Autodesk Fusion 360 part; units mm, degrees
sketch "Sketch2" plane through (0, 0, 0) normal (0, 0, 1) x (1, 0, 0)
  line L0 (-21.3111, -3.5) -> (-24.01, -3.5)
  line L1 (-27.5, -0.01) -> (-27.5, 0.01)
  line L2 (-24.01, 3.5) -> (-21.3111, 3.5)
  line L3 (27.5, 0.01) -> (27.5, -0.01)
  arc A0 (-27.5, -0.01) -> (-24.01, -3.5) centre (-24.01, -0.01) ccw
  arc A1 (-24.01, 3.5) -> (-27.5, 0.01) centre (-24.01, 0.01) ccw
  arc A2 (27.5, 0.01) -> (24.01, 3.5) centre (24.01, 0.01) ccw
  arc A3 (24.01, -3.5) -> (27.5, -0.01) centre (24.01, -0.01) ccw
  circle A4 centre (24, 0) radius 2.5
  circle A5 centre (-24, 0) radius 2.5
  circle A6 centre (6.7175, 6.7175) radius 1.65
  circle A7 centre (-5.6569, 5.6569) radius 1.65
  circle A8 centre (-6.7175, -6.7175) radius 1.65
  circle A9 centre (5.6569, -5.6569) radius 1.65
  circle A10 centre (0, 0) radius 12.5
  line L4 (-17.9244, 4.3738) -> (-6.0478, 10.9396)
  line L5 (-17.9244, -4.3738) -> (-6.0478, -10.9396)
  line L6 (17.9244, 4.3738) -> (6.0478, 10.9396)
  line L7 (17.9244, -4.3738) -> (6.0478, -10.9396)
  arc A11 (-21.3111, 3.5) -> (-17.9244, 4.3738) centre (-21.3111, 10.5) ccw
  arc A12 (-17.9244, -4.3738) -> (-21.3111, -3.5) centre (-21.3111, -10.5) ccw
  line L8 (24.01, 3.5) -> (21.3111, 3.5)
  line L9 (24.01, -3.5) -> (21.3111, -3.5)
  arc A13 (21.3111, -3.5) -> (17.9244, -4.3738) centre (21.3111, -10.5) ccw
  arc A14 (17.9244, 4.3738) -> (21.3111, 3.5) centre (21.3111, 10.5) ccw
  line L10 (21.3111, -3.5) -> (12, -3.5)
  line L11 (-12, -3.5) -> (-21.3111, -3.5)
  line L12 (-21.3111, 3.5) -> (-12, 3.5)
  line L13 (12, 3.5) -> (21.3111, 3.5)
  line L14 (-16.3799, 2.0847) -> (-27.5, 3.5) construction
  line L15 (-27.5, -3.5) -> (-16.3799, -2.0847) construction
  line L16 (-12.4, -1.5782) -> (12.4, 1.5782) construction
  line L17 (25.3613, 3.2278) -> (27.5, 3.5) construction
  line L18 (27.5, -3.5) -> (25.3613, -3.2278) construction
  line L19 (12.4, -1.5782) -> (-12.4, 1.5782) construction
  circle A15 centre (-16.01, 0.01) radius 2.5
  circle A16 centre (16, 0) radius 2.5
  dimension "d42" = 9.5
  dimension "d44" = 8
  dimension "d45" = 8
  dimension "d46" = 9.5
  dimension "d47" = 55
  dimension "d48" = 7
  dimension "d49" = 3.49
  dimension "d50" = 3.49
  dimension "d51" = 3.49
  dimension "d52" = 3.49
  dimension "d53" = 24
  dimension "d54" = 5
  dimension "d55" = 24
  dimension "d56" = 5
  dimension "d61" = 3.3
  dimension "d62" = 3.3
  dimension "d63" = 3.3
  dimension "d64" = 3.3
  dimension "d65" = 25
  dimension "d66" = 7
  dimension "d67" = 7
  dimension "d68" = 7
  dimension "d69" = 7
  dimension "d92" = 8
  dimension "d93" = 8
  dimension "d94" = 5
  dimension "d95" = 5
extrude "Extrude1" add sketch "Sketch2" along normal blind 8 contours L0 L1 L2 A0 A1 A10 L11 L12 makes body 1
extrude "Extrude2" add sketch "Sketch2" along normal blind 8 separate body contours L3 A2 A3 A10 L8 L9 L10 L13 makes body 2
extrude "Extrude3" add sketch "Sketch2" along normal blind 3 separate body contours A10 L5 A12 L11 | A10 | A10 L4 A11 L12 | A10 L7 A13 L10 | A10 L6 A14 L13 makes body 3
sketch "Sketch3" plane through (0, 0, 0) normal (0, 0, 1) x (1, 0, 0)
  circle A0 centre (-15, 0) radius 3.1
  circle A1 centre (-24, 0) radius 3.1
  circle A2 centre (15, 0) radius 3.1
  circle A3 centre (24, 0) radius 3.1
  dimension "d76" = 6.2
  dimension "d77" = 6.2
  dimension "d78" = 6.2
  dimension "d79" = 6.2
extrude "Extrude4" cut sketch "Sketch3" along normal blind 1 contours A1 bodies 1
extrude "Extrude7" cut sketch "Sketch3" along normal blind 1 contours A3 bodies 2
chamfer "Chamfer1" distance 2 distance2 1 1 edges at (4.1185, -5.0602, 0) measured on face at (7.3048, -5.7391, 2) on bodies 3
chamfer "Chamfer2" distance 2 distance2 1 3 edges at (-8.2559, -6.1208, 0) (-7.1952, 6.2535, 0) (5.1792, 7.3142, 0) measured on face at (-5.0696, -6.7998, 2) measured on face at (-4.0089, 5.5746, 2) measured on face at (8.3655, 6.6353, 2) on bodies 3
extrude "Extrude8" cut sketch "Sketch2" along normal blind 10 contours A15 bodies 1
extrude "Extrude9" cut sketch "Sketch2" along normal blind 10 contours A16 bodies 2
sketch "Sketch4" plane through (0, 0, 0) normal (0, 0, 1) x (1, 0, 0)
  circle A0 centre (-16, 0) radius 3
  circle A1 centre (16, 0) radius 3
  dimension "d100" = 6
  dimension "d101" = 6
extrude "Extrude10" cut sketch "Sketch4" along normal blind 1 contours A0 bodies 1
extrude "Extrude11" cut sketch "Sketch4" along normal blind 1 contours A1 bodies 2
sketch "Sketch5" plane through (0, 0, 0) normal (0, 0, 1) x (1, 0, 0)
  line L0 (0, 0) -> (5.6569, 5.6569)
  line L1 (0, 0) -> (8, 0) construction
  line L2 (0, 0) -> (-5.6569, -5.6569)
  line L3 (0, 0) -> (6.7175, -6.7175)
  line L4 (0, 0) -> (-6.7175, 6.7175)
  circle A0 centre (-6.7175, 6.7175) radius 1.65
  circle A1 centre (6.7175, -6.7175) radius 1.65
  circle A2 centre (-5.6569, -5.6569) radius 1.65
  circle A3 centre (5.6569, 5.6569) radius 1.65
  dimension "d106" = 8
  dimension "d107" = 45
  dimension "d108" = 8
  dimension "d109" = 9.5
  dimension "d110" = 9.5
  dimension "d111" = 3.3
  dimension "d112" = 3.3
  dimension "d113" = 3.3
  dimension "d114" = 3.3
extrude "Extrude12" add sketch "Sketch2" along normal blind 3 contours A10 | A6 | A7 | A8 | A9 bodies 3 2 1
extrude "Extrude13" cut sketch "Sketch5" along normal blind 10 contours A2 bodies 3
extrude "Extrude14" cut sketch "Sketch5" along normal blind 10 contours A3 | A1 | A0 bodies 3
chamfer "Chamfer3" distance 1 distance2 2 4 edges at (-7.1952, -6.2535, 0) (5.1792, -7.3142, 0) (-8.2559, 6.1208, 0) (4.1185, 5.0602, 0) measured on face at (1.9475, -1.9853, 0) measured on face at (1.9475, -1.9853, 0) measured on face at (1.9475, -1.9853, 0) measured on face at (1.9475, -1.9853, 0) on bodies 3
sketch "Sketch6" plane through (0, 0, 8) normal (0, 0, 1) x (-1, 0, 0)
  circle A0 centre (16.01, -0.01) radius 2.5
  circle A1 centre (24, 0) radius 2.5
  arc A2 (24.01, -3.5) -> (27.5, -0.01) centre (24.01, -0.01) ccw
  line L0 (27.5, -0.01) -> (27.5, 0.01)
  arc A3 (27.5, 0.01) -> (24.01, 3.5) centre (24.01, 0.01) ccw
  line L1 (24.01, 3.5) -> (12, 3.5)
  arc A4 (12, -3.5) -> (12, 3.5) centre (0, 0) ccw
  line L2 (12, -3.5) -> (24.01, -3.5)
  circle A5 centre (-16, 0) radius 3
  circle A6 centre (-24, 0) radius 3
  circle A7 centre (16.01, -0.01) radius 3
  circle A8 centre (24.01, 0.01) radius 3
  dimension "d123" = 6
  dimension "d124" = 6
  dimension "d125" = 6
  dimension "d126" = 6
extrude "Extrude15" cut sketch "Sketch6" against normal blind 1 contours A6 bodies 3
extrude "Extrude16" cut sketch "Sketch6" against normal blind 1 contours A0 | A5 | A7 | A8 bodies 3
combine "Combine1" [suppressed]
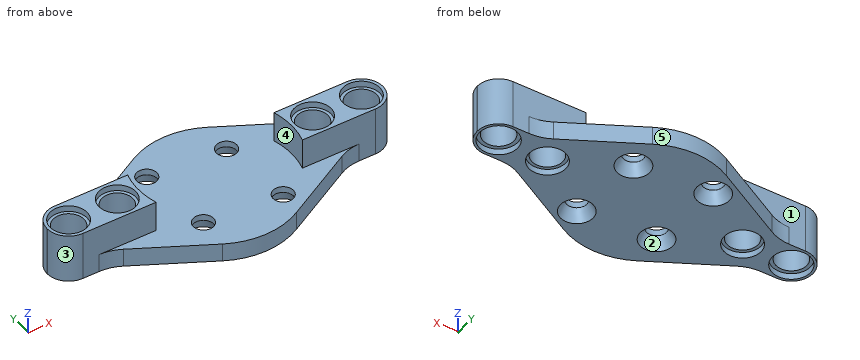
Could you check a few things on this model? Use its own coordinates, in mm. Face numbers are marked on the shaded views. A direction names the side the tool comes from. Coordinates: 2 decimals unless noted, no trailing zeros. Order: outer loops, then holes, each group sorted by start corner. A loop starts at its lowest first (then second) coordinate and runs counter-clockwise, first axis right, second up.
Q1. Please list where these lines run through material, in increasing order: L1, parallel to X at y = 0, z = 4.15; L2, parallel to Y at x = -16.01, z = 4.6; L3, parallel to X at y = 0.01, z = 7.6.
Q2. Suppose I cut it at C-C on x = -16. Please give me the cut outline in (y, z).
Q3. Suppose I cut it at A-A on z = 3.75. Give the number of separate pieces and of enclosed holes in the cut face, and give its area (3 significant figures).
Q4. Thinking about a two-plate mould opening in X: for the marked faces 1, 2 and 3, which applies, released by +X, released by -X, zero draft, split by the parting line, or undercut?
Q5. Will these pins go through, and if not, where does the flat tip stop? pin 1 (2.5 mm diameter, centred on x = 21, z = 5, fed in from +Y); pin 2 (2 mm diameter, centred on y = -2, z = 3.5, fed in from -X); pin 3 (2 mm diameter, centred on x = 6, y = 8, fed in from +Z); pin 4 (1 mm diameter, centred on x = -11, z = 4, fed in from +Y).
Q6. Suppose I cut it at D-D on x = 1. Please give me the cut outline in (y, z), and give its area (3 significant figures).
Q7. Suppose I cut it at B-B on x = 14. Please give me the cut outline in (y, z).
Q8. Which directions (+Z, -Z, +X, -X, +Y, -Y) give clear straight access to the entire face, cutting with the end or side of a thin tool? Please do the marked faces 4 and 5.
Answer:
1. L1: x = -27.5 to -26.5, -21.5 to -18.51, -13.51 to -12.5, 12.5 to 13.5, 18.5 to 21.5, 26.5 to 27.5
1. L2: y = -3.5 to -2.49, 2.51 to 3.5
1. L3: x = -27.5 to -27.01, -21.01 to -19.01, -13.01 to -12.5, 12.5 to 13, 19 to 21, 27 to 27.5
2. outline: (-5.44, 0) - (-3, 0) - (-3, 1) - (-2.49, 1) - (-2.49, 7) - (-2.99, 7) - (-2.99, 8) - (-3.5, 8) - (-3.5, 3) - (-5.44, 3) - close; (2.51, 1) - (3, 1) - (3, 0) - (5.44, 0) - (5.44, 3) - (3.5, 3) - (3.5, 8) - (3.01, 8) - (3.01, 7) - (2.51, 7) - close
3. separate pieces: 2
3. enclosed holes: 4
3. area: 123 mm2
4. face 1: zero draft
4. face 2: undercut
4. face 3: released by -X
5. pin 1: stops at y = 3.5
5. pin 2: stops at x = -27.36
5. pin 3: stops at z = 3
5. pin 4: passes through
6. outline: (-12.46, 0) - (12.46, 0) - (12.46, 3) - (-12.46, 3) - close
6. area: 74.8 mm2
7. outline: (-6.54, 0) - (-2.24, 0) - (-2.24, 1) - (-1.5, 1) - (-1.5, 7) - (-2.24, 7) - (-2.24, 8) - (-3.5, 8) - (-3.5, 3) - (-6.54, 3) - close; (1.5, 1) - (2.24, 1) - (2.24, 0) - (6.54, 0) - (6.54, 3) - (3.5, 3) - (3.5, 8) - (2.24, 8) - (2.24, 7) - (1.5, 7) - close
8. face 4: +Z
8. face 5: +Z, -Z, +Y
